```python
from build123d import *

# Parameters (mm, degrees)
SKETCH1_W           = 599
SKETCH1_H           = 599
BOSS_EXTRUDE1_DEPTH = 15
SKETCH2_R           = 5
CUT_EXTRUDE1_DEPTH  = 16
FILLET1_R           = 10
SKETCH3_R           = 35
CUT_EXTRUDE2_DEPTH  = 16
SKETCH4_R           = 3
CUT_EXTRUDE3_DEPTH  = 16
SKETCH5_R           = 2.1
CUT_EXTRUDE4_DEPTH  = 16


with BuildPart() as part:
    # Sketch1 → Boss-Extrude1 (new body)
    with BuildSketch(Plane.XY):
        Rectangle(SKETCH1_W, SKETCH1_H)
    extrude(amount=BOSS_EXTRUDE1_DEPTH)

    # Sketch2 → Cut-Extrude1 (cut, through all)
    with BuildSketch(Plane.XY.offset(15)):
        with Locations((-279.5, -279.5)):
            Circle(SKETCH2_R)
        with Locations((279.5, -279.5)):
            Circle(SKETCH2_R)
        with Locations((-279.5, 279.5)):
            Circle(SKETCH2_R)
        with Locations((279.5, 279.5)):
            Circle(SKETCH2_R)
        with Locations((279.5, 0)):
            Circle(SKETCH2_R)
    extrude(amount=-CUT_EXTRUDE1_DEPTH, mode=Mode.SUBTRACT)

    # Fillet1
    fillet1_edges = [part.edges().sort_by_distance(p)[0] for p in [
        (-299.5, -299.5, 7.5),
        (299.5, -299.5, 7.5),
        (-299.5, 299.5, 7.5),
        (299.5, 299.5, 7.5),
    ]]
    fillet(fillet1_edges, radius=FILLET1_R)

    # Sketch3 → Cut-Extrude2 (cut, through all)
    with BuildSketch(Plane.XY.offset(15)):
        with Locations((-180.79, -215.5)):
            Circle(SKETCH3_R)
    extrude(amount=-CUT_EXTRUDE2_DEPTH, mode=Mode.SUBTRACT)

    # Sketch4 → Cut-Extrude3 (cut, through all)
    with BuildSketch(Plane.XY.offset(15)):
        with Locations((-200, 170.5)):
            Circle(SKETCH4_R)
        with Locations((-200, 10.5)):
            Circle(SKETCH4_R)
        with Locations((200, 170.5)):
            Circle(SKETCH4_R)
        with Locations((200, 10.5)):
            Circle(SKETCH4_R)
        with Locations((138.4, -30.5)):
            Circle(SKETCH4_R)
        with Locations((-211.6, -30.5)):
            Circle(SKETCH4_R)
    extrude(amount=-CUT_EXTRUDE3_DEPTH, mode=Mode.SUBTRACT)

    # Sketch5 → Cut-Extrude4 (cut, through all)
    with BuildSketch(Plane.XY.offset(15)):
        with Locations((-224, 170.5)):
            Circle(SKETCH5_R)
        with Locations((224, 170.5)):
            Circle(SKETCH5_R)
        with Locations((224, 10.5)):
            Circle(SKETCH5_R)
        with Locations((201.236161147, -92.982459034)):
            Circle(SKETCH5_R)
        with Locations((178.85, -275.5)):
            Circle(SKETCH5_R)
        with Locations((-231.95, -275.5)):
            Circle(SKETCH5_R)
        with Locations((-249.6, -30.5)):
            Circle(SKETCH5_R)
        with Locations((-224, 10.5)):
            Circle(SKETCH5_R)
        with Locations((176.4, -30.5)):
            Circle(SKETCH5_R)
    extrude(amount=-CUT_EXTRUDE4_DEPTH, mode=Mode.SUBTRACT)


solid = part.part
```
Here's how the part is built. I have some questions about the finished solid (model axes, mm). Coordinates: 2 decimals unless noted, no trailing zeros. Order: outer loops, then holes, each group sorted by start corner. A loop starts at its lowest first (then second) coordinate and runs counter-clockwise, first axis right, second up. Notation, with made-up numbers: M 56.25,52 L 71.25,52 A15 cw 71.25,66 Z; hole C 38.5,28 d10. An arc over 180 degrees is marked long. Answer as a JSON object with one key per item and string values. Group by question number.
(1) Suppose I cut it at A-A, the plane y = -215.5. Please give me the cut outline in (x, z), then the cut area to 4 significant figures.
(2) For pin 1 (5.5 mm diameter, centred on x = 201.24, y = -92.98, fed in from -Z); pin 2 (2.5 mm diameter, centred on x = 176.4, y = -30.5, fed in from +Z), each with a flat end and sliding along its axis, tell me the tip position at first contact or that it passes through.
(3) I need wall thicknesses on probe 1 along Y at (x, z) = (-279.5, 4.75); probe 2 along X at (y, z) = (170.5, 9); probe 3 along Y at (x, z) = (279.5, 10.25). Which ranges of each line are inside material? Lowest first, please.
(4) If we mould it in two halves opening along Y, with no side actions, what happens to faces 1 (the face through (-147.406, -204.987, 7.605)), 2 (the face through (-4, 299.5, 7)), 3 (the face through (-4, -299.5, 7)), 4 (the face through (-299.5, -4, 7))? For each: released by +Y, released by -Y, zero draft, split by the parting line, or undercut.
Values found:
{
 "1": {"outline": "M -299.5,0 L -215.79,0 L -215.79,15 L -299.5,15 Z; M -145.79,0 L 299.5,0 L 299.5,15 L -145.79,15 Z", "area": "7,935 mm^2"},
 "2": {"pin 1": "stops at z = 0", "pin 2": "passes through"},
 "3": {"probe 1": "y = -299.5 to -284.5, -274.5 to 274.5, 284.5 to 299.5", "probe 2": "x = -299.5 to -226.1, -221.9 to -203, -197 to 197, 203 to 221.9, 226.1 to 299.5", "probe 3": "y = -299.5 to -284.5, -274.5 to -5, 5 to 274.5, 284.5 to 299.5"},
 "4": {"face 1": "undercut", "face 2": "released by +Y", "face 3": "released by -Y", "face 4": "zero draft"}
}
